```python
from build123d import *

# Parameters (mm, degrees)
SKETCH1_W           = 40
SKETCH1_H           = 30
BOSS_EXTRUDE1_DEPTH = 20
CHAMFER1_SIZE2      = 2.99999902
CHAMFER1_SIZE       = 3


with BuildPart() as part:
    # Sketch1 → Boss-Extrude1 (new body)
    with BuildSketch(Plane(origin=(0, 0, 0), x_dir=(1, 0, 0), z_dir=(0, 1, 0))):
        Rectangle(SKETCH1_W, SKETCH1_H)
    extrude(amount=BOSS_EXTRUDE1_DEPTH)

    # Chamfer1
    chamfer1_edges = [part.edges().sort_by_distance(p)[0] for p in [
        (20, 20, 0),
        (0, 20, -15),
        (-20, 20, 0),
        (0, 0, -15),
        (20, 0, 0),
        (0, 0, 15),
        (-20, 0, 0),
        (-20, 10, -15),
        (20, 10, -15),
        (20, 10, 15),
        (-20, 10, 15),
        (0, 20, 15),
    ]]
    chamfer(chamfer1_edges, length=CHAMFER1_SIZE, length2=CHAMFER1_SIZE2)


solid = part.part
```
Verification items for the finished model (mm, model axes). Coordinates: 2 decimals unless noted, no trailing zeros. Loops run counter-clockwise (first coordinate to the right, second up) from the corner with the lowest first, then second, coordinate; pieces in that order, holes last. Notation, with made-up numbers: (-32, 62) - (-20, 62) arc R11 cw to (-20, 71) - close; hole circle Ø2 at (71.5, 50.5). An arc over 180 degrees is marked (long way). Answer as a JSON object with one key per item and string values.
(1) Cross-section at B-B, the plane z = 11. Record the boundary of the cut face in (x, y).
Response:
{"outline": "(-20, 3) - (-17, 0) - (17, 0) - (20, 3) - (20, 17) - (17, 20) - (-17, 20) - (-20, 17) - close"}
(2) Scan lines: line 1 along X through (y, z) = (17.25, 7.25); line 2 along Y through (x, z) = (-3, 12.25); line 3 along X through (y, z) = (1.5, -10.75). Record each from-to range of solid material in increasing order.
Response:
{"line 1": "x = -19.75 to 19.75", "line 2": "y = 0.25 to 19.75", "line 3": "x = -18.5 to 18.5"}
(3) Cross-section at A-A, the plane x = 15. Record the boundary of the cut face in (y, z).
Response:
{"outline": "(0, -12) - (3, -15) - (17, -15) - (20, -12) - (20, 12) - (17, 15) - (3, 15) - (0, 12) - close"}
